Part model, mm, in its own coordinate system. Round coordinates to 2 decimals unless told otherwise and drop trailing zeros. Write each loop counter-clockwise with the first axis right and the second up, starting at its lowest first coordinate (ties: lowest second). Pieces come first, ordered by that corner, then holes. Notation, with made-up numbers: (-12, 15) -> (-4, 15) arc R36 ccw to (-4, 50) -> close; hole circle Ø5 at (80.25, -21.5). An arc over 180 degrees is marked (long way). Return JSON: item names as keys, results as strings. Group by question number.
(1) Drop flat-ended pins along their axis: pin 1 Ø13 at (x, z) = (12, 403.5) entering from +Y; pin 2 Ø12 at (y, z) = (14, 293) entering from +X. Give the stop position or say it passes through.
(2) Drill centre lines: L1, parallel to Y at x = 6.25, z = 836.5; L2, parallel to X at y = 9, z = 903; L3, parallel to Y at x = 1, z = 694. Where is each one in solid material? Low to high. Write a range as from..to.
(3) Saw through at A-A (z = 895.5). List the corners of the cut face in (x, y), plus the area to 3 significant figures.
(4) Saw through at B-B (x = 12.5). List the corners of the cut face in (y, z), plus the area to 3 significant figures.
(5) Saw through at C-C (y = 16). List the corners of the cut face in (x, z).
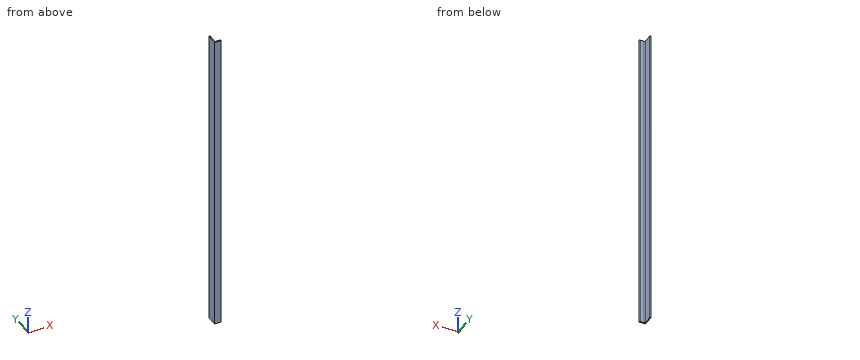
Autodesk Inventor part; units mm, degrees
ref_plane "Start Plane" through (0, 0, 0) normal (0, 0, 1) x (1, 0, 0)
ref_plane "End Plane" through (0, 0, 1400) normal (0, 0, 1) x (1, 0, 0)
ref_plane "YZ Plane" through (0, 0, 0) normal (1, 0, 0) x (0, 1, 0)
ref_plane "Start Plane" through (0, 0, 0) normal (0, 0, 1) x (1, 0, 0)
ref_plane "End Plane" through (0, 0, 1400) normal (0, 0, 1) x (1, 0, 0)
sketch "Sketch" plane through (0, 0, 0) normal (0, 0, 1) x (1, 0, 0)
  line L0 (-2.41, 28.7) -> (-2.41, -7.3)
  line L1 (-7.41, 32.7) -> (-6.41, 32.7)
  line L2 (-7.41, -17.3) -> (-7.41, 32.7)
  line L3 (22.59, -17.3) -> (-7.41, -17.3)
  line L4 (22.59, -16.3) -> (22.59, -17.3)
  line L5 (2.59, -12.3) -> (18.59, -12.3)
  arc A0 (-2.41, -7.3) -> (2.59, -12.3) centre (2.59, -7.3) ccw
  arc A1 (-2.41, 28.7) -> (-6.41, 32.7) centre (-6.41, 28.7) ccw
  arc A2 (22.59, -16.3) -> (18.59, -12.3) centre (18.59, -16.3) ccw
  line L6 (0, 43.6941) -> (0, -27.4657) construction
  line L7 (-13.5757, 0) -> (29.5841, 0) construction
  point P0 (-2.41, 32.7)
  point P1 (-2.41, -12.3)
  point P2 (22.59, -12.3)
  dimension "d4" = 30
  dimension "d6" = 50
  dimension "d8" = 5
  dimension "d10" = 5
  dimension "d17" = 5
  dimension "d18" = 4
  dimension "d19" = 17.3
  dimension "d20" = 7.41
extrude "Body" add sketch "Sketch" along normal up to surface (1400 mm away) from surface at 0
sketch "Sketch3" plane through (0, 0, 0) normal (0, 0, 1) x (1, 0, 0)
  line L0 (0, 0) -> (10, 0)
ref_plane "Work Plane10" through (0, 0, 0) normal (0, -1, 0) x (1, 0, 0)
sketch "Sketch4" plane through (0, 0, 0) normal (0, -1, 0) x (1, 0, 0)
  line L0 (-2, 0) -> (12, 0)
  line L1 (-2, 1400) -> (12, 1400)
  dimension "d24" = 1400
equation "\"d4\" = b"
equation "\"d6\" = ParH"
equation "\"d17\" = R"
equation "\"d18\" = R1"
equation "\"d19\" = ex"
equation "\"d20\" = ey"
equation "\"d11\" = G_L"
equation "\"b\" = 30"
equation "\"ParT\" = 5"
equation "\"R1\" = 4"
equation "\"G_L\" = d24"
equation "\"ParH\" = 50"
equation "\"R\" = 5"
equation "\"ey\" = 7.41"
equation "\"ex\" = 17.3"
equation "\"G_OFFSET_START\" = 0"
equation "\"G_OFFSET_END\" = 0"
properties part number "ISO 657-2 - 50x 30x 5-1400" material "Steel, Mild"
Computed values:
{
 "1": {"pin 1": "y = -12.3", "pin 2": "x = -2.41"},
 "2": {"L1": "-17.3..-12.3", "L2": "-7.41..-2.41", "L3": "-17.3..-12.04"},
 "3": {"outline": "(-7.41, -17.3) -> (22.59, -17.3) -> (22.59, -16.3) arc R4 ccw to (18.59, -12.3) -> (2.59, -12.3) arc R5 cw to (-2.41, -7.3) -> (-2.41, 28.7) arc R4 ccw to (-6.41, 32.7) -> (-7.41, 32.7) -> close", "area": "373 mm2"},
 "4": {"outline": "(-17.3, 0) -> (-12.3, 0) -> (-12.3, 1400) -> (-17.3, 1400) -> close", "area": "7,000 mm2"},
 "5": {"outline": "(-7.41, 0) -> (-2.41, 0) -> (-2.41, 1400) -> (-7.41, 1400) -> close"}
}
